Could you check a few things on this drawing? It's one solid part, dimensions in mm from its lowest x, y, z. A direction names the side the tool comes from. Round coordinates to 2 decimals unless told otherwise and drop trailing zeros. Write each loop counter-clockwise with the first axis right and the second up, starting at its lowest first coordinate (ties: lowest second). Pieces come first, ordered by that corner, then holes. Notation, with made-up numbers: (40, 24) - (60, 24) arc R22 cw to (60, 52) - close; hole circle Ø9 at (5.25, -39.5). An arc over 180 degrees is marked (long way). Put each result on its own line as item: value.
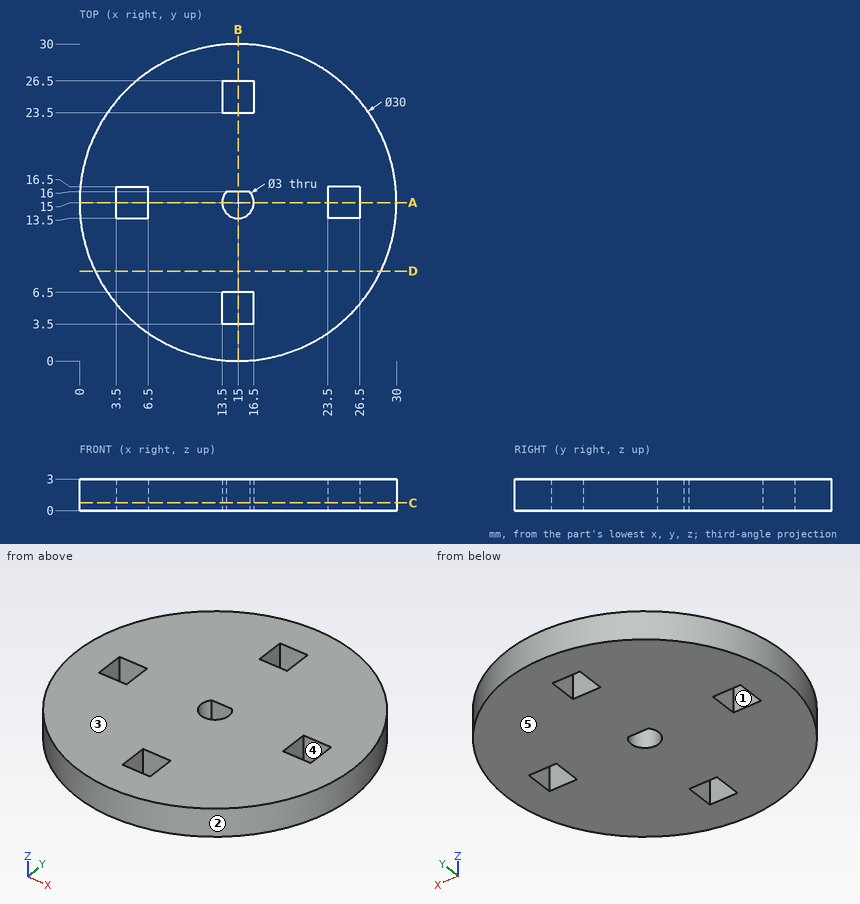
(1) Imagine slicing it at B-B, the plane x = 15. List the corners of the cut face in (y, z) for me, then the cut area to 3 significant figures.
Values found:
outline: (0, 0) - (3.5, 0) - (3.5, 3) - (0, 3) - close; (6.5, 0) - (13.5, 0) - (13.5, 3) - (6.5, 3) - close; (16, 0) - (23.5, 0) - (23.5, 3) - (16, 3) - close; (26.5, 0) - (30, 0) - (30, 3) - (26.5, 3) - close
area: 64.5 mm^2
(2) Imagine slicing it at A-A, the plane y = 15. List the corners of the cut face in (x, z) for me.
Values found:
outline: (0, 0) - (3.5, 0) - (3.5, 3) - (0, 3) - close; (6.5, 0) - (13.5, 0) - (13.5, 3) - (6.5, 3) - close; (16.5, 0) - (23.5, 0) - (23.5, 3) - (16.5, 3) - close; (26.5, 0) - (30, 0) - (30, 3) - (26.5, 3) - close
(3) If we mould it in two halves opening along X, with no side actions, what happens to the marked faces 1, 2 and 3? For each: pulls with the +X half, pulls with the -X half, needs draft (parallel to the pull), parting line crosses it, or undercut.
Values found:
face 1: undercut
face 2: parting line crosses it
face 3: needs draft
(4) For the marked faces 4 and 5, which set-ups out of +Z, -Z, +X, -X, +Y, -Y let a thin tool reach every point of the face, with its end or its side?
Values found:
face 4: +Z, -Z
face 5: -Z, +X, -X, +Y, -Y
(5) I'm going to push flat-ended pins straight in: pin 1 (1.5 mm diameter, centred on x = 5.5, z = 1, fed in from -Y); pin 2 (0.9 mm diameter, centred on y = 5, z = 1, fed in from +X); pin 3 (1.5 mm diameter, centred on x = 25.5, z = 1, fed in from -Y); pin 4 (1.8 mm diameter, centred on x = 15, y = 15, fed in from +Z). Where does each tip first touch, or does it pass through?
Values found:
pin 1: stops at y = 2.82
pin 2: stops at x = 26.57
pin 3: stops at y = 3.6
pin 4: passes through
(6) Imagine slicing it at C-C, the plane z = 0.75. List the corners of the cut face in (x, y) for me, then the cut area to 3 significant figures.
Values found:
outline: circle Ø30 at (15, 15); hole (3.5, 13.5) - (6.5, 13.5) - (6.5, 16.5) - (3.5, 16.5) - close; hole (13.5, 3.5) - (16.5, 3.5) - (16.5, 6.5) - (13.5, 6.5) - close; hole (13.5, 23.5) - (16.5, 23.5) - (16.5, 26.5) - (13.5, 26.5) - close; hole (13.88, 16) arc R1.5 ccw (long way) to (16.12, 16) - close; hole (23.5, 13.5) - (26.5, 13.5) - (26.5, 16.5) - (23.5, 16.5) - close
area: 665 mm^2
(7) Please list where these lines run through material, in increasing order: probe 1 along Y at (x, z) = (14.25, 1.8); probe 2 along X at (y, z) = (14.5, 2.15); probe 3 along Y at (x, z) = (16, 1.8). Write a range as from..to.
Values found:
probe 1: y = 0.02..3.5, 6.5..13.7, 16..23.5, 26.5..29.98
probe 2: x = 0.01..3.5, 6.5..13.59, 16.41..23.5, 26.5..29.99
probe 3: y = 0.03..3.5, 6.5..13.88, 16..23.5, 26.5..29.97
(8) Imagine slicing it at D-D, the plane y = 8.5. List the corners of the cut face in (x, z) for me.
Values found:
outline: (1.48, 0) - (28.52, 0) - (28.52, 3) - (1.48, 3) - close
